The drawing under review shows one solid part. Ordinate dimensions are in mm from its lowest x, y, z. A direction names the side the tool comes from. Round coordinates to 2 decimals unless told otherwise and drop trailing zeros. Loops run counter-clockwise (first coordinate to the right, second up) from the corner with the lowest first, then second, coordinate; pieces in that order, holes last. Notation, with made-up numbers: (-3, 82) -> (1, 82) arc R9 cw to (1, 87) -> close; hole circle Ø6 at (23.5, 49). An arc over 180 degrees is marked (long way). Use a Markdown table: item, result. Add a question column.
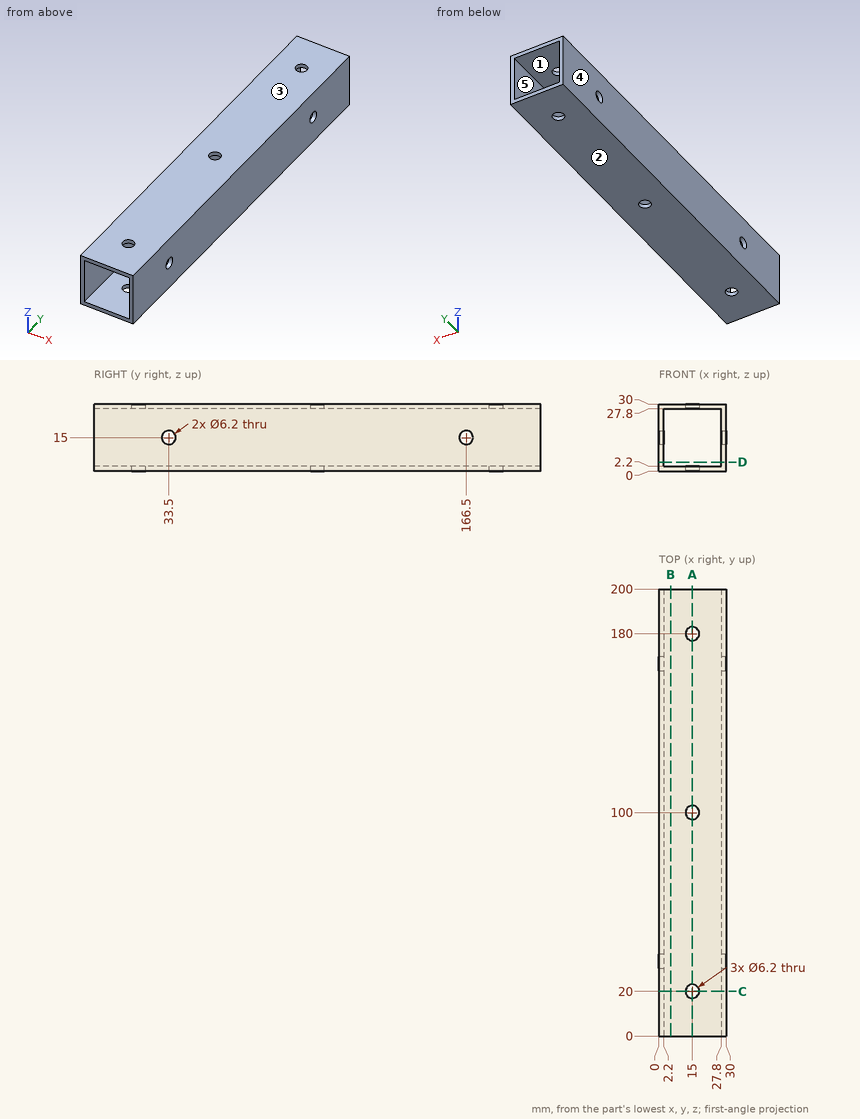
1. Consider section D-D on z = 4. State the section outline as (x, y) points.
2. Consider section C-C on y = 20. State the section outline as (x, z) points, plus the area to 3 significant figures.
3. Mouldability with a two-part tool opening along Z and no side actions: class the marked faces 3, 4 and 5 as +Z half, -Z half, draft (parallel to the pull), parting line (faces both ways), or undercut.
4. Consider section A-A on x = 15. Give the number of separate pieces and of enclosed holes in the cut face, plus the area to 3 significant figures.
5. Consider section B-B on x = 5.25. State the section outline as (y, z) points, plus the area to 3 significant figures.
6. To check wall thickness, follow probe 1 along Y at (x, z) = (15, 0.5); probe 2 along X at (y, z) = (147, 11.25); probe 3 along X at (y, z) = (20, 29.4). State the ranges of each line that lie inside material, in increasing order. Write a range as from..to.
7. For the marked faces 1 and 2, list the 3-axis set-ups (+Z, -Z, +X, -X, +Y, -Y) from which the entire face can be reached by the end or side of a thin tool; tool diameter is ignored.
Verdict:
| question | item | result |
|---|---|---|
| 1 | outline | (0, 0) -> (2.2, 0) -> (2.2, 200) -> (0, 200) -> close; (27.8, 0) -> (30, 0) -> (30, 200) -> (27.8, 200) -> close |
| 2 | outline | (0, 0) -> (11.9, 0) -> (11.9, 2.2) -> (2.2, 2.2) -> (2.2, 27.8) -> (11.9, 27.8) -> (11.9, 30) -> (0, 30) -> close; (18.1, 0) -> (30, 0) -> (30, 30) -> (18.1, 30) -> (18.1, 27.8) -> (27.8, 27.8) -> (27.8, 2.2) -> (18.1, 2.2) -> close |
| 2 | area | 217 mm² |
| 3 | face 3 | +Z half |
| 3 | face 4 | draft |
| 3 | face 5 | undercut |
| 4 | separate pieces | 8 |
| 4 | enclosed holes | 0 |
| 4 | area | 798 mm² |
| 5 | outline | (0, 0) -> (200, 0) -> (200, 2.2) -> (0, 2.2) -> close; (0, 27.8) -> (200, 27.8) -> (200, 30) -> (0, 30) -> close |
| 5 | area | 880 mm² |
| 6 | probe 1 | y = 0..16.9, 23.1..96.9, 103.1..176.9, 183.1..200 |
| 6 | probe 2 | x = 0..2.2, 27.8..30 |
| 6 | probe 3 | x = 0..11.9, 18.1..30 |
| 7 | face 1 | +Y, -Y |
| 7 | face 2 | -Z, +X, -X, +Y, -Y |
